Job drawing, mm, ordinate dimensions from the low corner. One solid piece. A direction names the side the tool comes from. Round coordinates to 2 decimals unless told otherwise and drop trailing zeros. Loops run counter-clockwise (first coordinate to the right, second up) from the corner with the lowest first, then second, coordinate; pieces in that order, holes last.
1) Band-saw the part on B-B, the plane z = 3. Write the cut outline in (x, y).
2) Drop flat-ended pins along their axis: P1, Ø4, axis at x = 34, z = 72.5, coming from the +Y side; P2, Ø2.5, axis at x = 33, y = 6, coming from the +Z side; P3, Ø5.5, axis at y = 3.5, z = 45, coming from the +X side. Give the stop position or say it passes through.
3) Band-saw the part on A-A, the plane x = 87. Write the cut outline in (y, z).
4) Band-saw the part on C-C, the plane x = 45. Write the cut outline in (y, z).
5) Probe line 1 (X direction, y = 0.55, z = 3); line 2 (X direction, y = 1, z = 72.5); line 3 (Z direction, x = 44, y = 1.25). List the from-to ranges inside material, lowest first.
6) 3-axis set-ups, long thin cutter, end or side, ignore diameter. For the marked faces 1 and 2: which of +Z, -Z, +X, -X, +Y, -Y reach the whole face in a straight line?
7) Band-saw the part on D-D, the plane z = 54.5. Write the cut outline in (x, y).
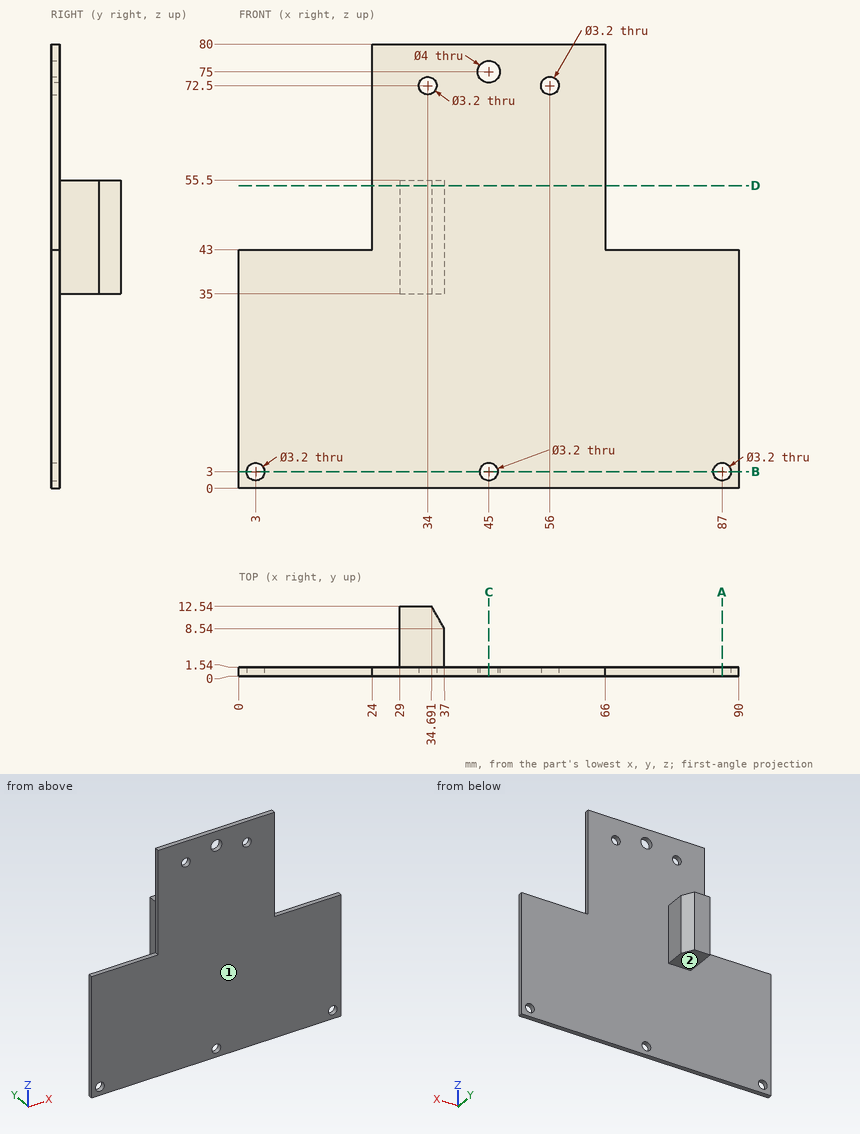
Reported:
1. outline: (0, 0) - (1.4, 0) - (1.4, 1.54) - (0, 1.54) - close; (4.6, 0) - (43.4, 0) - (43.4, 1.54) - (4.6, 1.54) - close; (46.6, 0) - (85.4, 0) - (85.4, 1.54) - (46.6, 1.54) - close; (88.6, 0) - (90, 0) - (90, 1.54) - (88.6, 1.54) - close
2. P1: stops at y = 1.54
2. P2: stops at z = 55.5
2. P3: stops at x = 66
3. outline: (0, 0) - (1.54, 0) - (1.54, 1.4) - (0, 1.4) - close; (0, 4.6) - (1.54, 4.6) - (1.54, 43) - (0, 43) - close
4. outline: (0, 0) - (1.54, 0) - (1.54, 1.4) - (0, 1.4) - close; (0, 4.6) - (1.54, 4.6) - (1.54, 73) - (0, 73) - close; (0, 77) - (1.54, 77) - (1.54, 80) - (0, 80) - close
5. line 1: x = 0 to 1.4, 4.6 to 43.4, 46.6 to 85.4, 88.6 to 90
5. line 2: x = 24 to 32.4, 35.6 to 54.4, 57.6 to 66
5. line 3: z = 0 to 1.75, 4.25 to 73.27, 76.73 to 80
6. face 1: +Z, -Z, +X, -X, -Y
6. face 2: -Z, +X, -X, +Y
7. outline: (24, 0) - (66, 0) - (66, 1.54) - (37, 1.54) - (37, 8.54) - (34.69, 12.54) - (29, 12.54) - (29, 1.54) - (24, 1.54) - close
